```python
from build123d import *

# Parameters (mm, degrees)
EXTRUDE_THIN1_DEPTH = 12.7
CUT_EXTRUDE1_DEPTH  = 55.111973556
SKETCH3_R           = 3.81
CUT_EXTRUDE2_DEPTH  = 54.488360816


with BuildPart() as part:
    # Sketch1 → Extrude-Thin1 (new, symmetric)
    with BuildSketch(Plane.XY):
        with BuildLine():
            Line((-44.45, -0.4191), (-3.666174209, -0.4191))
            ThreePointArc((-3.666174209, -0.4191), (-0.700724209, -1.213689933), (1.470135858, -3.38455))
            Line((1.470135858, -3.38455), (15.512048753, -27.70585657))
            Line((15.512048753, -27.70585657), (16.237951247, -27.28675657))
            Line((16.237951247, -27.28675657), (2.196038351, -2.96545))
            ThreePointArc((2.196038351, -2.96545), (-0.281624209, -0.487787439), (-3.666174209, 0.4191))
            Line((-3.666174209, 0.4191), (-44.45, 0.4191))
            Line((-44.45, 0.4191), (-44.45, -0.4191))
        make_face()
    extrude(amount=EXTRUDE_THIN1_DEPTH, both=True)

    # Sketch2 → Cut-Extrude1 (cut, through all)
    with BuildSketch(Plane(origin=(0, 0.4191, 0), x_dir=(1, 0, 0), z_dir=(0, 1, 0))):
        with BuildLine():
            Line((-34.689149884, 4.399409051), (-29.609149884, 4.399409051))
            ThreePointArc((-29.609149884, 4.399409051), (-27.069149884, 0), (-29.609149884, -4.399409051))
            Line((-29.609149884, -4.399409051), (-34.689149884, -4.399409051))
            ThreePointArc((-34.689149884, -4.399409051), (-37.229149884, 0), (-34.689149884, 4.399409051))
        make_face()
    extrude(amount=-CUT_EXTRUDE1_DEPTH, mode=Mode.SUBTRACT)

    # Sketch3 → Cut-Extrude2 (cut, through all)
    with BuildSketch(Plane(origin=(-0.362951247, -0.20955, 0), x_dir=(0, 0, 1), z_dir=(-0.8660254037844389, -0.49999999999999983, 0))):
        with Locations(Location((0, -19.05, 0), (0, 0, 270))):
            Circle(SKETCH3_R)
    extrude(amount=-CUT_EXTRUDE2_DEPTH, mode=Mode.SUBTRACT)


solid = part.part
```
Work out the finished part from the listing and answer in its coordinate system (mm). A direction names the side the tool comes from. Coordinates: 2 decimals unless noted, no trailing zeros. Loops run counter-clockwise (first coordinate to the right, second up) from the corner with the lowest first, then second, coordinate; pieces in that order, holes last.
1) Section A-A (x = -31) is taken. Give the vertices of the cut face in (y, z), plus the area to 3 significant figures.
Results:
outline: (-0.42, -12.7) - (0.42, -12.7) - (0.42, -4.4) - (-0.42, -4.4) - close; (-0.42, 4.4) - (0.42, 4.4) - (0.42, 12.7) - (-0.42, 12.7) - close
area: 13.9 mm2
2) Section B-B (z = 1.5) is taken. Give the vertices of the cut face in (x, y).
Results:
outline: (-44.45, -0.42) - (-37, -0.42) - (-37, 0.42) - (-44.45, 0.42) - close; (-27.3, -0.42) - (-3.67, -0.42) arc R5.93 cw to (1.47, -3.38) - (7.41, -13.67) - (8.14, -13.26) - (2.2, -2.97) arc R6.77 ccw to (-3.67, 0.42) - (-27.3, 0.42) - close; (10.91, -19.74) - (15.51, -27.71) - (16.24, -27.29) - (11.64, -19.32) - close
3) For faces 4 (the cylindrical face through (-0.74, -1.19, 0.18)), 5 (the cylindrical face through (-27.07, 0.01, -0.07)), determine the directions among +Z, -Z, +X, -X, +Y, -Y from which every point of the face is accessible in a straight line to the end or side of a thin tool.
Results:
face 4: +Z, -Z, -X, -Y
face 5: +Y, -Y
4) Section C-C (z = 5) is taken. Give the vertices of the cut face in (x, y).
Results:
outline: (-44.45, -0.42) - (-3.67, -0.42) arc R5.93 cw to (1.47, -3.38) - (15.51, -27.71) - (16.24, -27.29) - (2.2, -2.97) arc R6.77 ccw to (-3.67, 0.42) - (-44.45, 0.42) - close
5) Section D-D (x = -18) is taken. Give the vertices of the cut face in (y, z).
Results:
outline: (-0.42, -12.7) - (0.42, -12.7) - (0.42, 12.7) - (-0.42, 12.7) - close
6) Flat-ended cylindrical pins translate along their axes: pin 1 (12 mm diameter, centred on x = -9, z = 9.5, fed in from -Y); pin 2 (10 mm diameter, centred on y = -11, z = 0, fed in from -X); pin 3 (3 mm diameter, centred on y = -6, z = 9.5, fed in from -X). Find the tip coordinate at first contact, or state that the pin passes through.
Results:
pin 1: stops at y = -0.46
pin 2: stops at x = 2.98
pin 3: stops at x = 2.11
7) Consider probe 1 along Y at (x, z) = (-28.5, -10.25); probe 2 along Y at (x, z) = (7, 8); probe 3 along X at (y, z) = (-24.75, 0). Determine where each line is inside the solid, lowest interval first.
Results:
probe 1: y = -0.42 to 0.42
probe 2: y = -12.96 to -11.29
probe 3: x = 13.81 to 14.77
8) For a pull along Z with two mould halves and no side action, classify faces 1 (the flat face through (-12, 0, -12.7)), 2 (the cylindrical face through (-37.23, 0.01, 0.07)), 3 (the flat face through (-24, -0.419, 0)) as +Z half, -Z half, draft (parallel to the pull), parting line (faces both ways), or undercut.
Results:
face 1: -Z half
face 2: undercut
face 3: draft
